Geometry: final body of the model. Coordinates: model frame, mm. Face numbers are marked on the shaded views. Give positions to 0.01 mm unless a question says otherwise; leave off trailing zeros. Loops run counter-clockwise (first coordinate to the right, second up) from the corner with the lowest first, then second, coordinate; pieces in that order, holes last.
from build123d import *

# Parameters (mm, degrees)
CYLINDER027_R     = 2.5
CYLINDER027_DEPTH = 10
CYLINDER020_R     = 5
CYLINDER020_DEPTH = 5
CYLINDER019_R     = 5
CYLINDER019_DEPTH = 5
BOX005_W          = 15
BOX005_H          = 2
BOX005_DEPTH      = 20
FILLET002_R       = 2
BOX002_W          = 10
BOX002_H          = 2
BOX002_DEPTH      = 20
BOX_W             = 80
BOX_H             = 39
BOX_DEPTH         = 25
CYLINDER002_R     = 31.75
CYLINDER002_DEPTH = 25
BOX001_W          = 7.7
BOX001_H          = 7.7
BOX001_DEPTH      = 10
BOX007_W          = 72
BOX007_H          = 42
BOX007_DEPTH      = 2
CYLINDER_R        = 31.75
CYLINDER_DEPTH    = 18
CYLINDER001_R     = 34.5
CYLINDER001_DEPTH = 20
FILLET001_R       = 2
BOX006_W          = 15
BOX006_H          = 2
BOX006_DEPTH      = 20
FILLET003_R       = 2
CYLINDER026_R     = 3.5
CYLINDER026_DEPTH = 20


with BuildPart() as cylinder027:
    # Cylinder027 → Cylinder027 (new body)
    with BuildSketch(Plane(origin=(0, 33.25, 0), x_dir=(1, 0, 0), z_dir=(0, 0, 1))):
        Circle(CYLINDER027_R)
    extrude(amount=CYLINDER027_DEPTH)


with BuildPart() as cylinder020:
    # Cylinder020 → Cylinder020 (new body)
    with BuildSketch(Plane(origin=(-39.01, -14.6034, 15), x_dir=(1, 0, 0), z_dir=(0, 0, 1))):
        Circle(CYLINDER020_R)
    extrude(amount=CYLINDER020_DEPTH)


with BuildPart() as fusion013:
    # Cylinder019 → Cylinder019 (new body)
    with BuildSketch(Plane(origin=(38.99, -14.6034, 15), x_dir=(1, 0, 0), z_dir=(0, 0, 1))):
        Circle(CYLINDER019_R)
    extrude(amount=CYLINDER019_DEPTH)

    # Fusion013: union Cylinder020
    add(cylinder020.part)


with BuildPart() as fillet002:
    # Box005 → Box005 (new body)
    with BuildSketch(Plane(origin=(31.79, 6.35995, 0), x_dir=(1, 0, 0), z_dir=(0, 0, 1))):
        with Locations((7.5, 1)):
            Rectangle(BOX005_W, BOX005_H)
    extrude(amount=BOX005_DEPTH)

    # Fillet002
    fillet002_edges = [fillet002.edges().sort_by_distance(p)[0] for p in [
        (46.79, 7.35995, 20),
        (46.79, 7.35995, 0),
    ]]
    fillet(fillet002_edges, radius=FILLET002_R)


with BuildPart() as kostka002:
    # Box002 → Box002 (new body)
    with BuildSketch(Plane(origin=(31.22162, 4.362905, 0), x_dir=(1, 0, 0), z_dir=(0, 0, 1))):
        with Locations((5, 1)):
            Rectangle(BOX002_W, BOX002_H)
    extrude(amount=BOX002_DEPTH)


with BuildPart() as kostka:
    # Box → Box (new body)
    with BuildSketch(Plane(origin=(-38, -32.5, 0), x_dir=(1, 0, 0), z_dir=(0, 0, 1))):
        with Locations((40, 19.5)):
            Rectangle(BOX_W, BOX_H)
    extrude(amount=BOX_DEPTH)


with BuildPart() as cut001:
    # Cylinder002 → Cylinder002 (new body)
    with BuildSketch(Plane.XY):
        Circle(CYLINDER002_R)
    extrude(amount=CYLINDER002_DEPTH)

    # Cut001: cut Kostka
    add(kostka.part, mode=Mode.SUBTRACT)


with BuildPart() as kostka001:
    # Box001 → Box001 (new body)
    with BuildSketch(Plane(origin=(25.1, -7, 10), x_dir=(0, 1, 0), z_dir=(0, 0, 1))):
        with Locations((3.85, 3.85)):
            Rectangle(BOX001_W, BOX001_H)
    extrude(amount=BOX001_DEPTH)


with BuildPart() as kostka007:
    # Box007 → Box007 (new body)
    with BuildSketch(Plane(origin=(-36.01, -35.6034, 18), x_dir=(1, 0, 0), z_dir=(0, 0, 1))):
        with Locations((36, 21)):
            Rectangle(BOX007_W, BOX007_H)
    extrude(amount=BOX007_DEPTH)


with BuildPart() as cylinder:
    # Cylinder → Cylinder (new body)
    with BuildSketch(Plane.XY):
        Circle(CYLINDER_R)
    extrude(amount=CYLINDER_DEPTH)


with BuildPart() as fusion001:
    # Cylinder001 → Cylinder001 (new body)
    with BuildSketch(Plane.XY):
        Circle(CYLINDER001_R)
    extrude(amount=CYLINDER001_DEPTH)

    # Cut: cut Cylinder
    add(cylinder.part, mode=Mode.SUBTRACT)

    # Fusion: union Kostka007
    add(kostka007.part)

    # Cut002: cut Kostka001
    add(kostka001.part, mode=Mode.SUBTRACT)

    # Cut003: cut Cut001
    add(cut001.part, mode=Mode.SUBTRACT)

    # Cut004: cut Kostka002
    add(kostka002.part, mode=Mode.SUBTRACT)

    # Fillet001
    fillet001_edges = [fusion001.edges().sort_by_distance(p)[0] for p in [
        (-36.01, -35.6034, 19),
        (35.99, -35.6034, 19),
    ]]
    fillet(fillet001_edges, radius=FILLET001_R)

    # Fusion001: union Fillet002
    add(fillet002.part)


with BuildPart() as cut015:
    # Box006 → Box006 (new body)
    with BuildSketch(Plane(origin=(31.7936, 2.359946, 0), x_dir=(1, 0, 0), z_dir=(0, 0, 1))):
        with Locations((7.5, 1)):
            Rectangle(BOX006_W, BOX006_H)
    extrude(amount=BOX006_DEPTH)

    # Fillet003
    fillet003_edges = [cut015.edges().sort_by_distance(p)[0] for p in [
        (46.7936, 3.359946, 20),
        (46.7936, 3.359946, 0),
    ]]
    fillet(fillet003_edges, radius=FILLET003_R)

    # Fusion002: union Fusion001
    add(fusion001.part)

    # Cut015: cut Fusion013
    add(fusion013.part, mode=Mode.SUBTRACT)


with BuildPart() as base:
    # Cylinder026 → Cylinder026 (new body)
    with BuildSketch(Plane(origin=(0, 35.25, 0), x_dir=(1, 0, 0), z_dir=(0, 0, 1))):
        Circle(CYLINDER026_R)
    extrude(amount=CYLINDER026_DEPTH)

    # Fusion019: union Cut015
    add(cut015.part)

    # Cut023: cut Cylinder027
    add(cylinder027.part, mode=Mode.SUBTRACT)


solid = base.part
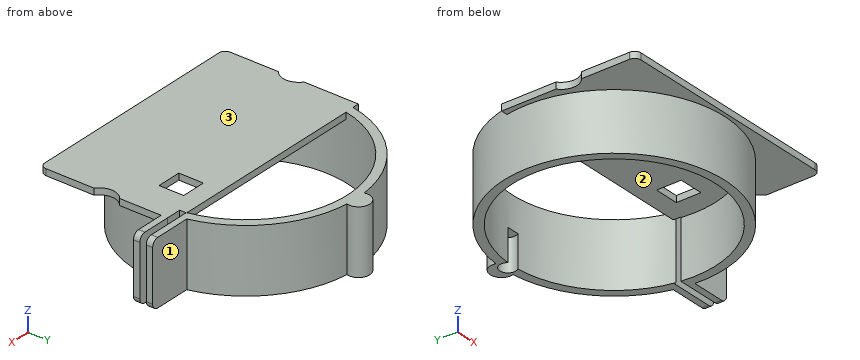
Item 1: Section query A-A on x = 0. Return loops of the section in (y, z).
Values follow:
outline: (-35.6, 18) - (-34.5, 18) - (-34.5, 0) - (-31.75, 0) - (-31.75, 18) - (6.5, 18) - (6.5, 20) - (-35.6, 20) - close; (31.75, 10) - (35.75, 10) - (35.75, 0) - (38.75, 0) - (38.75, 20) - (31.75, 20) - close
Item 2: Ray query, probe 1 along Y at (x, z) = (0, 6.5); probe 2 along X at (y, z) = (0, 13); probe 3 along Z at (x, y) = (-17, -6). Return the intervals inside material, ascending.
Values follow:
probe 1: y = -34.5 to -31.75, 35.75 to 38.75
probe 2: x = -34.5 to -31.75, 31.75 to 34.5
probe 3: z = 18 to 20
Item 3: Section query D-D on y = 33.25. Return loops of the section in (x, z).
Values follow:
outline: (-9.2, 0) - (-2.5, 0) - (-2.5, 10) - (2.5, 10) - (2.5, 0) - (9.2, 0) - (9.2, 20) - (-9.2, 20) - close
Item 4: Pin query (flat end, axial travel): pin 1 (6 mm diameter, centred on x = 0, y = 33.25, fed in from -Z); pin 2 (4 mm diameter, centred on y = -8.5, z = 4, fed in from +X); pin 3 (12 mm diameter, centred on x = -5.5, y = 0.5, fed in from -Z); pin 4 (0.6 mm diameter, centred on x = 31.5, z = 14, fed in from -Y). Return the tip coordinate at first contact, or that it passes through.
Values follow:
pin 1: stops at z = 0
pin 2: stops at x = 33.88
pin 3: stops at z = 18
pin 4: stops at y = -14.72
Item 5: Section query B-B on y = 19. Return loops of the section in (x, z).
Values follow:
outline: (-28.8, 0) - (-25.44, 0) - (-25.44, 20) - (-28.8, 20) - close; (25.44, 0) - (28.8, 0) - (28.8, 20) - (25.44, 20) - close
Item 6: Draft query along Y for the marked faces 1, 2 and 3. Return one class per face: +Y half, -Y half, draft (parallel to the pull), parting line (faces both ways), or undercut.
Values follow:
face 1: +Y half
face 2: undercut
face 3: draft
